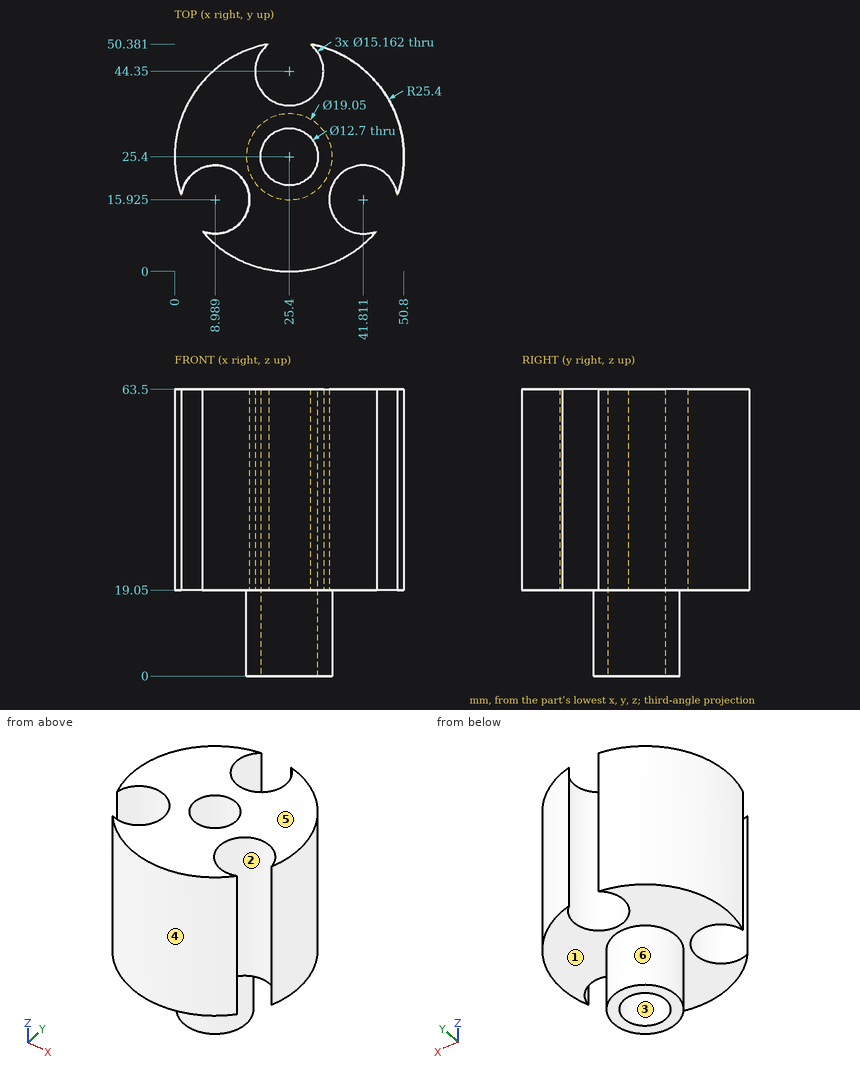
Could you check a few things on this drawing? It's one solid part, dimensions in mm from its lowest x, y, z. A direction names the side the tool comes from. Give positions to 0.01 mm unless a question says otherwise; leave off trailing zeros. Write item = value, one per line.
(1) For the marked faces 5 and 6, which set-ups out of +Z, -Z, +X, -X, +Y, -Y let a thin tool reach every point of the face, with its end or its side?
Worked out:
face_5 = +Z, +X, -X, +Y, -Y
face_6 = -Z
(2) I'm going to push flat-ended pins straight in: P1, Ø3, axis at y = 14.5, z = 48, coming from the -X side; P2, Ø10, axis at x = 29, y = 6, coming from the -Z side; P3, Ø5, axis at y = 34, z = 54, coming from the -X side; P4, Ø7.5, axis at x = 25.4, y = 25.4, coming from the -Z side. Where does each tip first touch, or does it pass through?
Worked out:
P1 = 15.98
P2 = 19.05
P3 = 0.74
P4 = through
(3) Thinking about a two-plate mould opening in Y: for the marked faces 1, 2, 3 and 4, which applies, released by +Y, released by -Y, zero draft, split by the parting line, or undercut?
Worked out:
face_1 = zero draft
face_2 = undercut
face_3 = undercut
face_4 = released by -Y
(4) I need wall thicknesses on probe 1 along X at (y, z) = (25, 55.5); probe 2 along Y at (x, z) = (25, 40); probe 3 along Y at (x, z) = (25, 18.5). Which ranges of each line are inside material? Lowest first, please. Write a range as from..to.
Worked out:
probe_1 = 0..19.06, 31.74..50.8
probe_2 = 0..19.06, 31.74..36.78
probe_3 = 15.88..19.06, 31.74..34.92
